from build123d import *

# Parameters (mm, degrees)
F2_DEPTH = 500
F4_D     = 22
F4_DEPTH = 500
F4_TIP   = 6.6094668093


with BuildPart() as f2:
    # F1 (on Top) → F2 (new body)
    with BuildSketch(Plane.XY):
        with BuildLine():
            ThreePointArc((-163.0534820056, 70.1662666553), (-157.6223484782, 78.2824576852), (-155.7149531136, 87.8601197772))
            ThreePointArc((-155.7149531136, 87.8601197772), (-155.7191665297, 88.3190893279), (-155.7318053575, 88.7779041722))
            ThreePointArc((-155.7318053575, 88.7779041722), (-196.2865938282, 107.4183406948), (-187.2075438541, 63.7179105685))
            ThreePointArc((-187.2075438541, 63.7179105685), (-177.008627135, 63.1363832526), (-167.4285546343, 66.6829713514))
            ThreePointArc((-167.4285546343, 66.6829713514), (-165.1433123991, 68.3018988597), (-163.0534820056, 70.1662666553))
        make_face()
        with BuildLine():
            ThreePointArc((-167.4285546343, 66.6829713514), (-177.008627135, 63.1363832526), (-187.2075438541, 63.7179105685))
            Line((-187.2075438541, 63.7179105685), (-158.4206221982, -128.3106024335))
            ThreePointArc((-158.4206221982, -128.3106024335), (-148.8405496975, -124.7640143347), (-138.6416329785, -125.3455416506))
            Line((-138.6416329785, -125.3455416506), (-167.4285546343, 66.6829713514))
        make_face()
        with BuildLine():
            ThreePointArc((-138.6416329785, -125.3455416506), (-148.8405496975, -124.7640143347), (-158.4206221982, -128.3106024335))
            ThreePointArc((-158.4206221982, -128.3106024335), (-157.2346377204, -171.364221804), (-120.1342237189, -149.4877508594))
            ThreePointArc((-120.1342237189, -149.4877508594), (-120.346610419, -146.2359472222), (-120.9801618704, -143.0393947726))
            ThreePointArc((-120.9801618704, -143.0393947726), (-125.5760028014, -133.9161101448), (-133.437474442, -127.3928180386))
            ThreePointArc((-133.437474442, -127.3928180386), (-135.9821279087, -126.2232039632), (-138.6416329785, -125.3455416506))
        make_face()
        with BuildLine():
            ThreePointArc((30.9279478124, -22.0949328208), (23.0664761717, -15.5716407145), (18.4706352408, -6.4483560868))
            Line((18.4706352408, -6.4483560868), (-133.437474442, -127.3928180386))
            ThreePointArc((-133.437474442, -127.3928180386), (-125.5760028014, -133.9161101448), (-120.9801618704, -143.0393947726))
            Line((-120.9801618704, -143.0393947726), (30.9279478124, -22.0949328208))
        make_face()
        with BuildLine():
            ThreePointArc((67.6246970892, 0), (52.2023591813, 23.0926046355), (24.9632259812, 17.6938531219))
            ThreePointArc((24.9632259812, 17.6938531219), (19.3601501931, 9.1520958101), (17.6415493331, -0.917784395))
            ThreePointArc((17.6415493331, -0.917784395), (17.9009605645, -3.7063259786), (18.4706352408, -6.4483560868))
            ThreePointArc((18.4706352408, -6.4483560868), (23.0664761717, -15.5716407145), (30.9279478124, -22.0949328208))
            ThreePointArc((30.9279478124, -22.0949328208), (55.5200696716, -21.417501394), (67.6246970892, 0))
        make_face()
        with BuildLine():
            ThreePointArc((-155.7318053575, 88.7779041722), (-155.7191665297, 88.3190893279), (-155.7149531136, 87.8601197772))
            ThreePointArc((-155.7149531136, 87.8601197772), (-157.6223484782, 78.2824576852), (-163.0534820056, 70.1662666553))
            Line((-163.0534820056, 70.1662666553), (17.6415493331, -0.917784395))
            ThreePointArc((17.6415493331, -0.917784395), (19.3601501931, 9.1520958101), (24.9632259812, 17.6938531219))
            Line((24.9632259812, 17.6938531219), (-155.7318053575, 88.7779041722))
        make_face()
    extrude(amount=F2_DEPTH)

    # F4
    with Locations(Plane.XY.offset(500)):
        with Locations((-180.7149531136, 87.8601197772), (42.6246970892, 0), (-145.1342237189, -149.4877508594)):
            Hole(F4_D / 2, depth=F4_DEPTH)
            with Locations((0, 0, -(F4_DEPTH + F4_TIP / 2))):  # 118° drill point
                Cone(0, F4_D / 2, F4_TIP, mode=Mode.SUBTRACT)


solid = f2.part
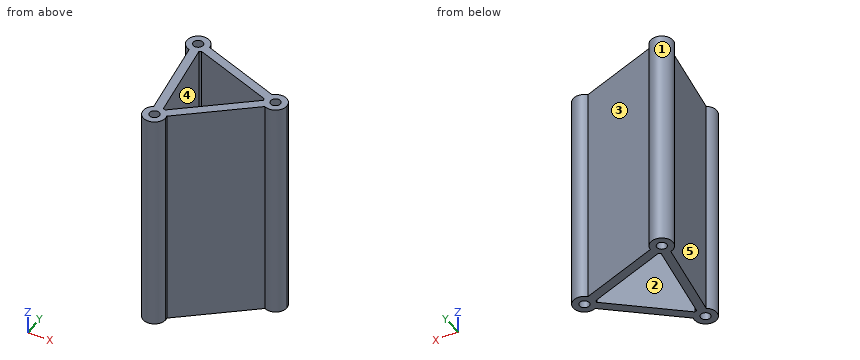
Design review of the part built by this model. Coordinates are the model's own, in mm. Face numbers are marked on the shaded views. A direction names the side the tool comes from. Round coordinates to 2 decimals unless told otherwise and drop trailing zeros. Write each loop counter-clockwise with the first axis right and the second up, starting at its lowest first coordinate (ties: lowest second). Pieces come first, ordered by that corner, then holes.
Item 1: For pin 1 Ø2 at (x, z) = (-157, 325.5) entering from +Y; pin 2 Ø6 at (y, z) = (-50.5, 354.5) entering from +X; pin 3 Ø5 at (y, z) = (-68.5, 381.5) entering from -X; pin 4 Ø1.5 at (x, y) = (-33.5, 32.5) entering from -Z, all flat-tipped, find the tip position at first contact; note any pin that passes through.
Item 2: For the marked faces 4 and 5, list the 3-axis set-ups (+Z, -Z, +X, -X, +Y, -Y) from which the entire face can be reached by the end or side of a thin tool; tool diameter is ignored.
Item 3: Draft analysis for pull direction Y (two halves, no side actions). For the marked faces 1, 2 and 3, state which applies: released by +Y, released by -Y, zero draft, split by the parting line, or undercut.
Item 4: Consider section B-B on z = 223. Give the boundary of the cut face in (x, y).
Item 5: Consider section C-C on x = -43.5. Give the boundary of the cut face in (y, z).
Item 6: Wall thickness on L1, parallel to X at y = -42.5, z = 366; L2, parallel to Y at x = -108, z = 168 (3 decimals); L3, parallel to Y at x = -127, z = 308.5: over which ranges is each line inside the solid? List them lowest first.
Item 7: Consider section A-A on y = 50. Give the boundary of the cut face in (x, z).
Check values:
1. pin 1: stops at y = 98.3
1. pin 2: stops at x = -0.98
1. pin 3: stops at x = -167.76
1. pin 4: stops at z = 0
2. face 4: +Z, -Z
2. face 5: +Z, -Z, -X
3. face 1: split by the parting line
3. face 2: undercut
3. face 3: released by +Y
4. outline: (-187.21, 63.72) - (-158.42, -128.31) arc R25 ccw (long way) to (-120.98, -143.04) - (30.93, -22.09) arc R25 ccw (long way) to (24.96, 17.69) - (-155.73, 88.78) arc R25 ccw (long way) to start; hole circle Ø22 at (-180.71, 87.86); hole (-167.43, 66.68) - (-138.64, -125.35) arc R25 cw to (-133.44, -127.39) - (18.47, -6.45) arc R25 cw to (17.64, -0.92) - (-163.05, 70.17) arc R25 cw to start; hole circle Ø22 at (-145.13, -149.49); hole circle Ø22 at (42.62, 0)
5. outline: (-81.35, 0) - (-55.79, 0) - (-55.79, 500) - (-81.35, 500) - close; (23.13, 0) - (44.63, 0) - (44.63, 500) - (23.13, 500) - close
6. L1: x = -171.28 to -151.06, -26.81 to 5.3
6. L2: y = -132.705 to -107.14, 48.509 to 70.001
6. L3: y = -166.7 to -122.27, 55.98 to 77.48
7. outline: (-185.15, 0) - (-164.93, 0) - (-164.93, 500) - (-185.15, 500) - close; (-111.79, 0) - (-57.16, 0) - (-57.16, 500) - (-111.79, 500) - close
